```python
from build123d import *

# Parameters (mm, degrees)
SKETCH_2_R               = 2.5
SKETCH_2_R_2             = 2.25
EXTRUDE_1_DEPTH          = 3
SKETCH_3_W               = 6
SKETCH_3_H               = 8
EXTRUDE_2_DEPTH          = 3.4
SKETCH_4_R               = 1.25
CUT_EXTRUDE_1_DEPTH      = 5
CUT_EXTRUDE_2_DEPTH      = 75.101012139
CUT_EXTRUDE_2_DEPTH_BACK = 3
SKETCH_5_R               = 1.75
CHAMFER_1_SIZE           = 1


with BuildPart() as part:
    # Эскиз2 → Бобышка-Вытянуть1 (new body)
    with BuildSketch(Plane.XY):
        with BuildLine():
            Line((-53, 35), (53, 35))
            ThreePointArc((53, 35), (61.485281374, 31.485281374), (65, 23))
            Line((65, 23), (65, -23))
            ThreePointArc((65, -23), (61.485281374, -31.485281374), (53, -35))
            Line((53, -35), (-53, -35))
            ThreePointArc((-53, -35), (-61.485281374, -31.485281374), (-65, -23))
            Line((-65, -23), (-65, 23))
            ThreePointArc((-65, 23), (-61.485281374, 31.485281374), (-53, 35))
        make_face()
        with Locations((10, -25)):
            Circle(SKETCH_2_R, mode=Mode.SUBTRACT)
        with Locations((25, -25)):
            Circle(SKETCH_2_R, mode=Mode.SUBTRACT)
        with Locations((40, -25)):
            Circle(SKETCH_2_R, mode=Mode.SUBTRACT)
        with Locations((-42.754119413, -25)):
            Circle(SKETCH_2_R_2, mode=Mode.SUBTRACT)
    extrude(amount=EXTRUDE_1_DEPTH)

    # Эскиз3 → Бобышка-Вытянуть2 (add)
    with BuildSketch(Plane(origin=(0, 0, 0), x_dir=(-1, 0, 0), z_dir=(0, 0, -1))):
        with Locations((0, -25)):
            Rectangle(SKETCH_3_W, SKETCH_3_H)
        with Locations((-50, -25)):
            Rectangle(SKETCH_3_W, SKETCH_3_H)
    extrude(amount=EXTRUDE_2_DEPTH)

    # Эскиз4 → Вырез-Вытянуть1 (cut)
    with BuildSketch(Plane(origin=(0, 0, -3.4), x_dir=(-1, 0, 0), z_dir=(0, 0, -1))):
        with Locations((-50, -25)):
            Circle(SKETCH_4_R)
        with Locations(Location((0, -25, 0), (0, 0, 180))):
            Circle(SKETCH_4_R)
    extrude(amount=-CUT_EXTRUDE_1_DEPTH, mode=Mode.SUBTRACT)

    # Эскиз5 → Вырез-Вытянуть2 (cut, two sides: drawn at the far end of the back side and taken through both)
    with BuildSketch(Plane.XY.offset(3).offset(-CUT_EXTRUDE_2_DEPTH_BACK)):
        with Locations(Location((-58.865243762, 28.354943792, 0), (0, 0, 180))):
            Circle(SKETCH_5_R)
        with Locations(Location((-58.865243762, -28.354943792, 0), (0, 0, 180))):
            Circle(SKETCH_5_R)
        with Locations(Location((58.865243762, 28.354943792, 0), (0, 0, 180))):
            Circle(SKETCH_5_R)
        with Locations(Location((58.865243762, -28.354943792, 0), (0, 0, 180))):
            Circle(SKETCH_5_R)
    extrude(amount=CUT_EXTRUDE_2_DEPTH + CUT_EXTRUDE_2_DEPTH_BACK, mode=Mode.SUBTRACT)

    # Фаска1
    chamfer_1_edges = [part.edges().sort_by_distance(p)[0] for p in [
        (-57.115243762, -28.354943792, 3),
        (60.615243762, 28.354943792, 3),
        (60.615243762, -28.354943792, 3),
        (-57.115243762, 28.354943792, 3),
    ]]
    chamfer(chamfer_1_edges, length=CHAMFER_1_SIZE)


solid = part.part
```
Geometry check sheet. Reference: the model listing, model coordinates, mm. A direction names the side the tool comes from. Coordinates: 2 decimals unless noted, no trailing zeros. Order: outer loops, then holes, each group sorted by start corner. A loop starts at its lowest first (then second) coordinate and runs counter-clockwise, first axis right, second up.
Item 1: Depth check by flat-ended pin: pin 1 (1 mm diameter, centred on y = -25, z = -2.5, fed in from -X); pin 2 (0.8 mm diameter, centred on x = 49.5, y = -25.5, fed in from -Z); pin 3 (1.7 mm diameter, centred on x = 49.5, z = -1, fed in from -Y). Enter the tip coordinate at first touch or a pass-through.
Item 2: Section check D-D (y = 2). Enter the section's corners in (x, z), plus the area to 3 significant figures.
Item 3: Scan lines: line 1 along Y through (x, z) = (50, -2.25); line 2 along X through (y, z) = (29.5, 2); line 3 along X through (y, z) = (-27.5, -2.25). Record each from-to range of solid material in increasing order.
Item 4: Section check C-C (x = 50). Enter the section's corners in (y, z), plus the area to 3 significant figures.
Item 5: Tool access check on faces 4 (the flat face through (0, -25, 1.6)), 5 (the flat face through (50, -29, -2)), 6 (the flat face through (1.4, -24.9, -3.4)), 7 (the flat face through (-3, -25, -2)), 8 (the flat face through (3, -25, -2)). Record the directions out of +Z, -Z, +X, -X, +Y, -Y that give a thin tool (end or side, any length) a straight path to the whole face; none if there is none.
Item 6: Section check A-A (z = -1). Enter the section's corners in (x, y), plus the area to 3 significant figures.
Item 7: Mould release check, pull along X, two halves, no side actions. Record for faces 1 (the flat face through (-1, 35, 1)), 2 (the flat face through (53, -25, -2)), 3 (the flat face through (47, -25, -2)): released by +X, released by -X, zero draft, split by the parting line, or undercut.
Item 8: Section check B-B (x = 25). Enter the section's corners in (y, z).
Check sheet entries:
1. pin 1: stops at x = -3
1. pin 2: stops at z = 1.6
1. pin 3: stops at y = -29
2. outline: (-65, 0) - (65, 0) - (65, 3) - (-65, 3) - close
2. area: 390 mm2
3. line 1: y = -29 to -26.25, -23.75 to -21
3. line 2: x = -63.09 to -60.19, -57.54 to 57.54, 60.19 to 63.09
3. line 3: x = -3 to 3, 47 to 53
4. outline: (-35, 0) - (-29, 0) - (-29, -3.4) - (-26.25, -3.4) - (-26.25, 1.6) - (-23.75, 1.6) - (-23.75, -3.4) - (-21, -3.4) - (-21, 0) - (35, 0) - (35, 3) - (-35, 3) - close
4. area: 225 mm2
5. face 4: -Z
5. face 5: -Z, +X, -X, -Y
5. face 6: -Z, +X, -X, +Y, -Y
5. face 7: -Z, -X, +Y, -Y
5. face 8: -Z, +Y, -Y
6. outline: (-3, -29) - (3, -29) - (3, -21) - (-3, -21) - close; (47, -29) - (53, -29) - (53, -21) - (47, -21) - close; hole circle Ø2.5 at (0, -25); hole circle Ø2.5 at (50, -25)
6. area: 86.2 mm2
7. face 1: zero draft
7. face 2: released by +X
7. face 3: undercut
8. outline: (-35, 0) - (-27.5, 0) - (-27.5, 3) - (-35, 3) - close; (-22.5, 0) - (35, 0) - (35, 3) - (-22.5, 3) - close
